```python
from build123d import *

# Parameters (mm, degrees)
SKETCH2_W           = 72
SKETCH2_H           = 30
SKETCH2_R           = 2.25
SKETCH2_R_2         = 1.6875
BOSS_EXTRUDE1_DEPTH = 10
SKETCH3_W           = 30
SKETCH3_H           = 30
SKETCH3_R           = 2.25
BOSS_EXTRUDE2_DEPTH = 4
FILLET1_R           = 2
FILLET2_R           = 2


with BuildPart() as part:
    # Sketch2 → Boss-Extrude1 (new body)
    with BuildSketch(Plane(origin=(0, 0, 0), x_dir=(1, 0, 0), z_dir=(0, 1, 0))):
        Rectangle(SKETCH2_W, SKETCH2_H)
        with Locations(Location((0, 0, 0), (0, 0, 270))):
            Circle(SKETCH2_R, mode=Mode.SUBTRACT)
        with Locations(Location((-6.363961031, 6.363961031, 0), (0, 0, 270))):
            Circle(SKETCH2_R_2, mode=Mode.SUBTRACT)
        with Locations(Location((6.363961031, -6.363961031, 0), (0, 0, 270))):
            Circle(SKETCH2_R_2, mode=Mode.SUBTRACT)
        with Locations(Location((4.242640687, 4.242640687, 0), (0, 0, 270))):
            Circle(SKETCH2_R_2, mode=Mode.SUBTRACT)
        with Locations(Location((-4.242640687, -4.242640687, 0), (0, 0, 270))):
            Circle(SKETCH2_R_2, mode=Mode.SUBTRACT)
    extrude(amount=BOSS_EXTRUDE1_DEPTH)

    # Sketch3 → Boss-Extrude2 (add)
    with BuildSketch(Plane.ZY.offset(36)):
        with Locations((0, 5)):
            Rectangle(SKETCH3_W, SKETCH3_H)
        with Locations((-11.5, 16.5)):
            Circle(SKETCH3_R, mode=Mode.SUBTRACT)
        with Locations((-11.5, -6.5)):
            Circle(SKETCH3_R, mode=Mode.SUBTRACT)
        with Locations((11.5, -6.5)):
            Circle(SKETCH3_R, mode=Mode.SUBTRACT)
        with Locations((11.5, 16.5)):
            Circle(SKETCH3_R, mode=Mode.SUBTRACT)
    boss_extrude2 = extrude(amount=BOSS_EXTRUDE2_DEPTH)

    # Mirror1: Boss-Extrude2 across plane
    add(boss_extrude2.mirror(Plane(origin=(0, 0, 0), x_dir=(0, 0, 1), z_dir=(1, 0, 0))))

    # Fillet1
    fillet1_edges = [part.edges().sort_by_distance(p)[0] for p in [
        (-36, 10, 0),
        (-36, 0, 0),
        (36, 0, 0),
        (36, 10, 0),
    ]]
    fillet(fillet1_edges, radius=FILLET1_R)

    # Fillet2
    fillet2_edges = [part.edges().sort_by_distance(p)[0] for p in [
        (-38, 20, 15),
        (-38, 20, -15),
        (-38, -10, -15),
        (-38, -10, 15),
        (38, 20, -15),
        (38, 20, 15),
        (38, -10, 15),
        (38, -10, -15),
    ]]
    fillet(fillet2_edges, radius=FILLET2_R)


solid = part.part
```
Design review of the part built by this model. Coordinates are the model's own, in mm. A direction names the side the tool comes from. Give positions to 0.01 mm unless a question says otherwise; leave off trailing zeros. Write each loop counter-clockwise with the first axis right and the second up, starting at its lowest first coordinate (ties: lowest second). Pieces come first, ordered by that corner, then holes. Notation, with made-up numbers: (62.25, 82) - (121.25, 82) arc R20 ccw to (121.25, 89) - close; hole circle Ø2 at (59, -26). An arc over 180 degrees is marked (long way). Return JSON: item names as keys, results as strings. Group by question number.
(1) To check wall thickness, follow probe 1 along Y at (x, z) = (-38.2, -11.5); probe 2 along X at (y, z) = (-4.25, 0); probe 3 along X at (y, z) = (9.75, -5.75). State the ranges of each line that lie inside material, in increasing order.
(2) We need section A-A, the plane z = 0. Give the boundary of the cut face in (x, y), then the cut area to 3 significant figures.
(3) Machinability: for faces 4 (the cylindrical face through (-35.43, 10.6, -0.21)), 5 (the flat face through (38, -10, 0)), 6 (the flat face through (36, -6, 0)), which of the approach directions +Z, -Z, +X, -X, +Y, -Y give a long, thin tool a straight path to every point of the face, cutting with its end or side? Answer none if there is none.
(4) We need section D-D, the plane z = 11.5. Give the number of separate pieces and of enclosed holes in the cut face, then the cut area to 3 significant figures.
(5) Insertion check: pin 1 (12 mm diameter, centred on x = -27.5, z = 2.5, fed in from +Y); pin 2 (15 mm diameter, centred on x = 13.5, z = 0.5, fed in from -Y). Each pin has a flat end and moves straight along its axis. Give the tip position at first contact, or say it passes through.
(6) Mouldability with a two-part tool opening along X and no side actions: class faces 1 (the cylindrical face through (37.97, -4.98, 9.84)), 2 (the flat face through (-40, 5, 0)), 3 (the cylindrical face through (-35.4, -0.57, -0.21)) as +X half, -X half, draft (parallel to the pull), parting line (faces both ways), or undercut.
(7) We need section B-B, the plane x = 0. Give the boundary of the cut face in (y, z), then the cut area to 3 significant figures.
(8) We need section C-C, the plane y = -6.5. Give the boundary of the cut face in (x, z).
Reported:
{
 "1": {"probe 1": "y = -10 to -8.75, -4.25 to 14.25, 18.75 to 20", "probe 2": "x = -40 to -36, 36 to 40", "probe 3": "x = -40 to -7.94, -4.79 to 3.48, 5 to 40"},
 "2": {"outline": "(-40, -10) - (-36, -10) - (-36, -2) arc R2 cw to (-34, 0) - (-2.25, 0) - (-2.25, 10) - (-34, 10) arc R2 cw to (-36, 12) - (-36, 20) - (-40, 20) - close; (2.25, 0) - (34, 0) arc R2 cw to (36, -2) - (36, -10) - (40, -10) - (40, 20) - (36, 20) - (36, 12) arc R2 cw to (34, 10) - (2.25, 10) - close", "area": "918 mm2"},
 "3": {"face 4": "+Z, -Z, +Y", "face 5": "+Z, -Z, +X, -X, -Y", "face 6": "+Z, -Z, -Y"},
 "4": {"separate pieces": "5", "enclosed holes": "0", "area": "891 mm2"},
 "5": {"pin 1": "stops at y = 10", "pin 2": "stops at y = 0"},
 "6": {"face 1": "draft", "face 2": "-X half", "face 3": "undercut"},
 "7": {"outline": "(0, -15) - (10, -15) - (10, -2.25) - (0, -2.25) - close; (0, 2.25) - (10, 2.25) - (10, 15) - (0, 15) - close", "area": "255 mm2"},
 "8": {"outline": "(-40, -15) - (-36, -15) - (-36, -13.75) - (-40, -13.75) - close; (-40, -9.25) - (-36, -9.25) - (-36, 9.25) - (-40, 9.25) - close; (-40, 13.75) - (-36, 13.75) - (-36, 15) - (-40, 15) - close; (36, -15) - (40, -15) - (40, -13.75) - (36, -13.75) - close; (36, -9.25) - (40, -9.25) - (40, 9.25) - (36, 9.25) - close; (36, 13.75) - (40, 13.75) - (40, 15) - (36, 15) - close"}
}
